Study the drawing (mm; zero at the part's minimum x, y, z) and answer. A direction names the side the tool comes from. Coordinates: 2 decimals unless noted, no trailing zeros. Write each loop counter-clockwise with the first axis right and the second up, starting at its lowest first coordinate (ties: lowest second). Pieces come first, ordered by that corner, then holes. Notation, with made-up numbers: (45.25, 57.5) - (81.25, 57.5) arc R35 cw to (81.25, 95.5) - close; hole circle Ø11 at (2.25, 15). An arc over 180 degrees is marked (long way). One line per item, written item: value.
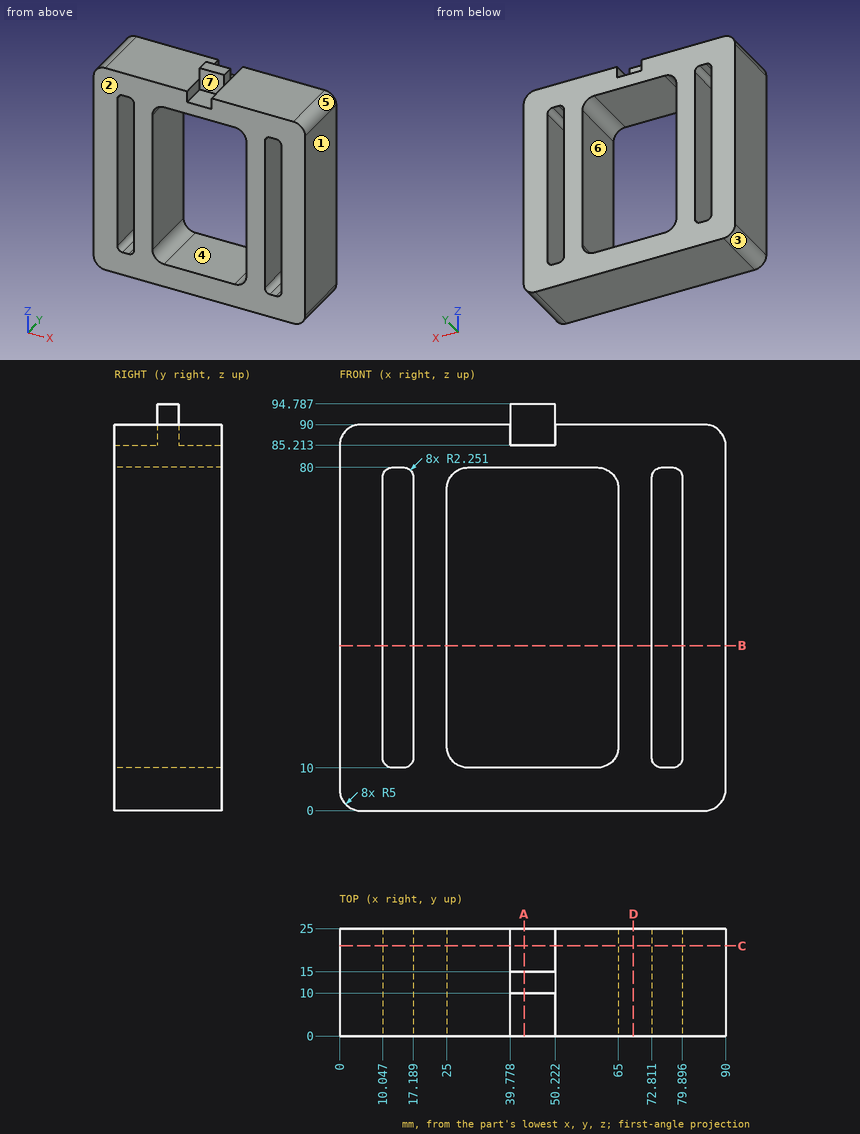
Item 1: Consider probe 1 along X at (y, z) = (18.5, 37.5); probe 2 along Z at (x, y) = (13.5, 8); probe 3 along X at (y, z) = (16.5, 77.5) (1 decimal). Determine where each line is inside the solid, lowest interval first.
Evaluation:
probe 1: x = 0 to 10.05, 17.19 to 25, 65 to 72.81, 79.9 to 90
probe 2: z = 0 to 10, 80 to 90
probe 3: x = 0 to 10, 17.2 to 25.7, 64.3 to 72.8, 79.9 to 90
Item 2: Which of the six approach directions +Z, -Z, +X, -X, +Y, -Y give full straight-line access (tool end or side, diameter ignored) to the marked faces 5, 6 and 7?
Evaluation:
face 5: +Z, +X, +Y, -Y
face 6: +Y, -Y
face 7: +Z, -Y
Item 3: Section B-B, the plane z = 38.5 is taken. Determine the outline of the cut face in (x, y).
Evaluation:
outline: (0, 0) - (10.05, 0) - (10.05, 25) - (0, 25) - close; (17.19, 0) - (25, 0) - (25, 25) - (17.19, 25) - close; (65, 0) - (72.81, 0) - (72.81, 25) - (65, 25) - close; (79.9, 0) - (90, 0) - (90, 25) - (79.9, 25) - close
Item 4: Section D-D, the plane x = 68.5 is taken. Determine the outline of the cut face in (y, z).
Evaluation:
outline: (0, 0) - (25, 0) - (25, 90) - (0, 90) - close
Item 5: Section C-C, the plane y = 21 is taken. Give the number of separate pieces and of enclosed holes in the cut face, then the cut area to 3 significant figures.
Evaluation:
separate pieces: 1
enclosed holes: 3
area: 4,260 mm2
Item 6: Section A-A, the plane x = 43 is taken. Determine the outline of the cut face in (y, z), then the cut area to 3 significant figures.
Evaluation:
outline: (0, 0) - (25, 0) - (25, 10) - (0, 10) - close; (0, 80) - (25, 80) - (25, 85.21) - (15, 85.21) - (15, 94.79) - (10, 94.79) - (10, 85.21) - (0, 85.21) - close
area: 428 mm2
Item 7: Determine the mould class of the marked faces 1, 2, 3 and 4 for opening direction X: +X half, -X half, draft (parallel to the pull), parting line (faces both ways), or undercut.
Evaluation:
face 1: +X half
face 2: draft
face 3: -X half
face 4: undercut
Item 8: Given pin 1 (1.4 mm diameter, centred on y = 19.5, z = 86.5, fed in from -X) (1 decimal); pin 2 (5 mm diameter, centred on x = 42.5, z = 90, fed in from +Y); pin 3 (1.4 mm diameter, centred on y = 11.5, z = 91.5, fed in from +X); pin 4 (4 mm diameter, centred on x = 15.5, z = 40.5, fed in from +Y), each flat-ended and moving along its own axis, determine where each tip first touches the part or whether it passes through.
Evaluation:
pin 1: stops at x = 0.1
pin 2: stops at y = 15
pin 3: stops at x = 50.22
pin 4: stops at y = 25
